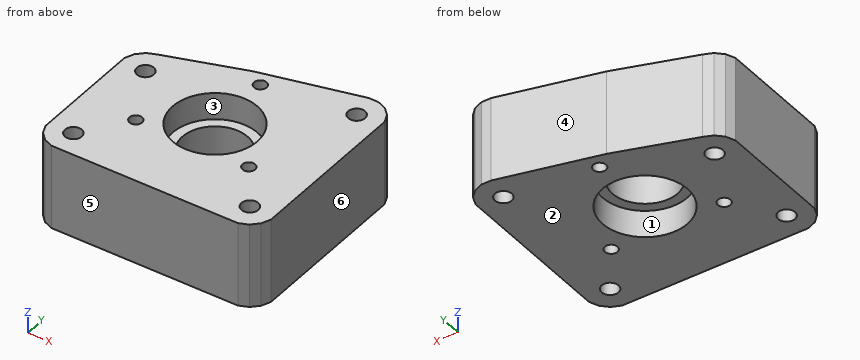
from build123d import *

# Parameters (mm, degrees)
CARTRIDGE_BODY_START    = 34
PROFILE_1_R             = 8.5
PROFILE_1_R_2           = 2.2
PROFILE_1_R_3           = 1.65
CARTRIDGE_BODY_DEPTH    = 22
INBOARD_608_SEAT_START  = 33.99
PROFILE_2_R             = 11.05
INBOARD_608_SEAT_DEPTH  = 7.01
OUTBOARD_608_SEAT_START = 49
PROFILE_3_R             = 11.05
OUTBOARD_608_SEAT_DEPTH = 7.01


with BuildPart() as part:
    # Profile_1 → Cartridge_body (new body)
    with BuildSketch(Plane.XY.offset(CARTRIDGE_BODY_START)):
        Polygon((-24.268087093, -26.375104323), (24.268087093, -26.375104323), (26.611206515, -25.40455248), (28.40455248, -23.611206515), (29.375104323, -21.268087093), (29.375104323, 21.268087093), (28.40455248, 23.611206515), (26.611206515, 25.40455248), (24.268087093, 26.375104323), (21.731912907, 26.375104323), (-3.999351601, 20.106098248), (-24.268087093, 13.375104323), (-26.611206515, 12.40455248), (-28.40455248, 10.611206515), (-29.375104323, 8.268087093), (-29.375104323, -21.268087093), (-28.40455248, -23.611206515), (-26.611206515, -25.40455248), align=None)
        Circle(PROFILE_1_R, mode=Mode.SUBTRACT)
        with Locations((-23, -20)):
            Circle(PROFILE_1_R_2, mode=Mode.SUBTRACT)
        with Locations((23, -20)):
            Circle(PROFILE_1_R_2, mode=Mode.SUBTRACT)
        with Locations((-23, 7)):
            Circle(PROFILE_1_R_2, mode=Mode.SUBTRACT)
        with Locations((23, 20)):
            Circle(PROFILE_1_R_2, mode=Mode.SUBTRACT)
        with Locations((0, 17)):
            Circle(PROFILE_1_R_3, mode=Mode.SUBTRACT)
        with Locations((-14.722431864, -8.5)):
            Circle(PROFILE_1_R_3, mode=Mode.SUBTRACT)
        with Locations((14.722431864, -8.5)):
            Circle(PROFILE_1_R_3, mode=Mode.SUBTRACT)
    extrude(amount=CARTRIDGE_BODY_DEPTH)

    # Profile_2 → Inboard_608_seat (cut)
    with BuildSketch(Plane.XY.offset(INBOARD_608_SEAT_START)):
        Circle(PROFILE_2_R)
    extrude(amount=INBOARD_608_SEAT_DEPTH, mode=Mode.SUBTRACT)

    # Profile_3 → Outboard_608_seat (cut)
    with BuildSketch(Plane.XY.offset(OUTBOARD_608_SEAT_START)):
        Circle(PROFILE_3_R)
    extrude(amount=OUTBOARD_608_SEAT_DEPTH, mode=Mode.SUBTRACT)


solid = part.part
Model file for the job. Use its own axes, mm. Face numbers are marked on the shaded views. A direction names the side the tool comes from. Give positions to 0.01 mm unless a question says otherwise; leave off trailing zeros. Loops run counter-clockwise (first coordinate to the right, second up) from the corner with the lowest first, then second, coordinate; pieces in that order, holes last. Notation, with made-up numbers: (-39, -19) -> (-17, -19) arc R14 cw to (-17, 3) -> close; hole circle Ø4 at (37.5, 32). An arc over 180 degrees is marked (long way). Use a Markdown table: item, result. Add a question column.
(1) Slice it at B-B on x = 23. List the corners of the cut face in (y, z), and give its area (3 significant figures).
(2) Mould opens along X. For the marked faces 3, 4, 5 and 6 say: +X half, -X half, draft (parallel to the pull), parting line (faces both ways), or undercut.
(3) Wall check: line 1 along Y through (x, z) = (21.5, 45.75); line 2 along Y through (x, z) = (0, 38.5); line 3 along X through (y, z) = (0, 54.5). Give the ranges that are in metal, low to high.
(4) Drop flat-ended pins along their axis: pin 1 Ø2.5 at (x, y) = (14.72, -8.5) entering from -Z; pin 2 Ø5.5 at (x, y) = (-14.72, -8.5) entering from +Z; pin 3 Ø11 at (x, y) = (3.5, -3.5) entering from -Z; pin 4 Ø2 at (y, z) = (9.5, 47) entering from -X. Give the stop position or say it passes through.
(5) Slice it at C-C on z = 53.5. Give the number of separate pieces and of enclosed holes in the cut face, and give its area (3 significant figures).
(6) Tool access for the marked faces 1 and 2: list every direction of +Z, -Z, +X, -X, +Y, -Y with a clear straight run to the whole face (end or side of a thin tool).
(7) Slice it at D-D on y = -18.5. List the corners of the cut face in (x, z), and give its area (3 significant figures).
(8) Slice it at A-A on y = 0. List the corners of the cut face in (x, z), and give its area (3 significant figures).
Filled sheet:
| question | item | result |
|---|---|---|
| 1 | outline | (-26.38, 34) -> (-22.2, 34) -> (-22.2, 56) -> (-26.38, 56) -> close; (-17.8, 34) -> (17.8, 34) -> (17.8, 56) -> (-17.8, 56) -> close; (22.2, 34) -> (26.38, 34) -> (26.38, 56) -> (22.2, 56) -> close |
| 1 | area | 967 mm2 |
| 2 | face 3 | undercut |
| 2 | face 4 | -X half |
| 2 | face 5 | draft |
| 2 | face 6 | +X half |
| 3 | line 1 | -26.38 to -21.61, -18.39 to 18.39, 21.61 to 26.32 |
| 3 | line 2 | -26.38 to -11.05, 11.05 to 15.35, 18.65 to 21.08 |
| 3 | line 3 | -29.38 to -11.05, 11.05 to 29.38 |
| 4 | pin 1 | through |
| 4 | pin 2 | z = 56 |
| 4 | pin 3 | z = 41 |
| 4 | pin 4 | x = -29.28 |
| 5 | separate pieces | 1 |
| 5 | enclosed holes | 8 |
| 5 | area | 2,250 mm2 |
| 6 | face 1 | -Z |
| 6 | face 2 | -Z, +X, -X, +Y, -Y |
| 7 | outline | (-29.38, 34) -> (-24.61, 34) -> (-24.61, 56) -> (-29.38, 56) -> close; (-21.39, 34) -> (21.39, 34) -> (21.39, 56) -> (-21.39, 56) -> close; (24.61, 34) -> (29.38, 34) -> (29.38, 56) -> (24.61, 56) -> close |
| 7 | area | 1,150 mm2 |
| 8 | outline | (-29.38, 34) -> (-11.05, 34) -> (-11.05, 41) -> (-8.5, 41) -> (-8.5, 49) -> (-11.05, 49) -> (-11.05, 56) -> (-29.38, 56) -> close; (8.5, 41) -> (11.05, 41) -> (11.05, 34) -> (29.38, 34) -> (29.38, 56) -> (11.05, 56) -> (11.05, 49) -> (8.5, 49) -> close |
| 8 | area | 847 mm2 |
